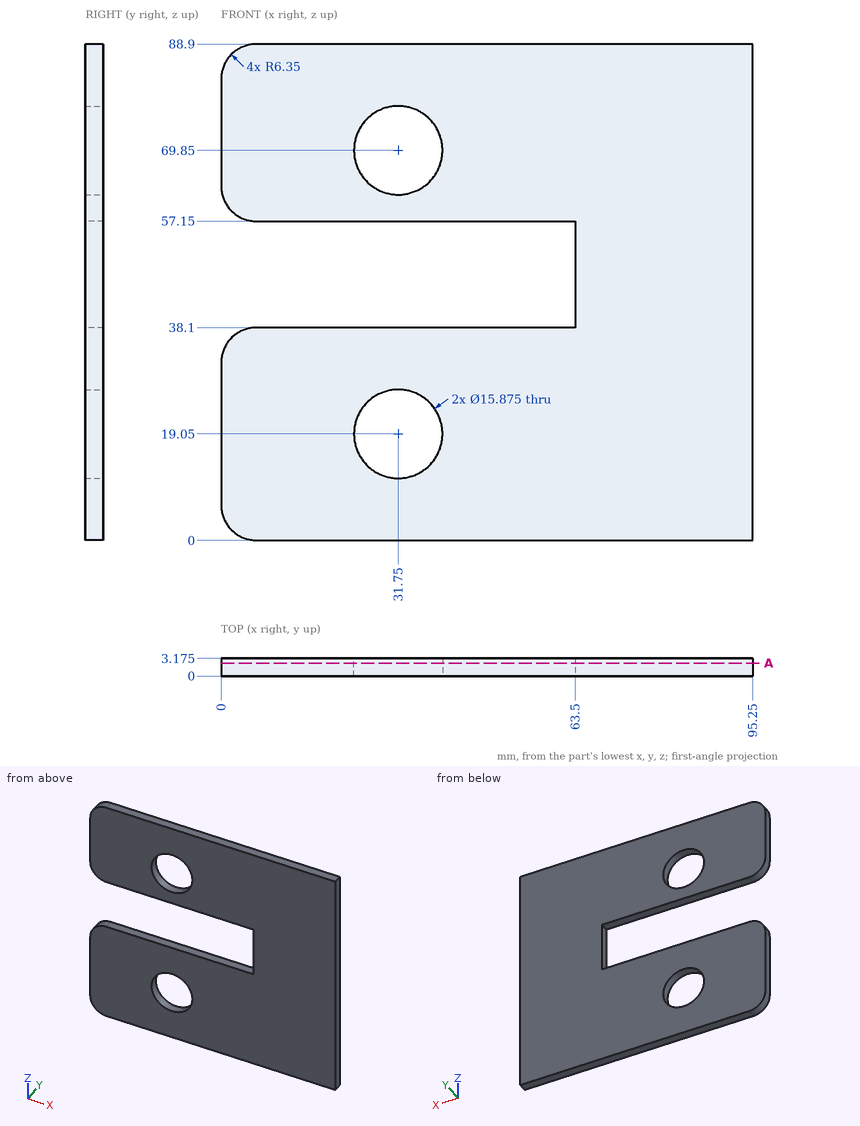
The figure shows three views and two pictorial views of one solid part (mm, origin at its lowest corner). Answer the questions. Give positions to 0.01 mm unless a question says otherwise; leave off trailing zeros. Write each question's results on one line, items separated by ' | '.
Q1. Section A-A, the plane y = 2.3 is taken. Count the separate pieces of the cut face and the enclosed holes in it, then the cut area to 3 significant figures.
Output values:
separate pieces: 1 | enclosed holes: 2 | area: 6,830 mm2
Q2. Consider L1, parallel to Z at x = 31.75, y = 2.5; L2, parallel to Z at x = 35.5, y = 0.4; L3, parallel to Z at x = 7, y = 2.45. Determine where each line is inside the solid, lowest interval first. Write a range as from..to.
Output values:
L1: 0..11.11, 26.99..38.1, 57.15..61.91, 77.79..88.9 | L2: 0..12.05, 26.05..38.1, 57.15..62.85, 76.85..88.9 | L3: 0..38.1, 57.15..88.9
Q3. Flat-ended cylindrical pins translate along their axes: P1, Ø14.5, axis at x = 31.75, z = 69.85, coming from the +Y side; P2, Ø1, axis at y = 1, z = 46, coming from the -X side. Find the tip coordinate at first contact, or state that the pin passes through.
Output values:
P1: through | P2: x = 63.5
